from build123d import *
from build123d import SkipClean  # not in build123d's __all__

# Parameters (mm, degrees)
F1_DEPTH = 51
F2_DEPTH = 90


with BuildPart() as f1:
    # F0 (on Front) → F1 (new body)
    with BuildSketch(Plane.XZ):
        with BuildLine():
            Line((1.45, 0.9), (2.0621590627, 0.9))
            ThreePointArc((2.0621590627, 0.9), (1.5909902577, 1.5909902577), (0.9, 2.0621590627))
            Line((0.9, 2.0621590627), (0.9, 1.45))
            Line((0.9, 1.45), (0, 1.45))
            Line((0, 1.45), (-0.9, 1.45))
            Line((-0.9, 1.45), (-0.9, 2.0621590627))
            ThreePointArc((-0.9, 2.0621590627), (-1.5909902577, 1.5909902577), (-2.0621590627, 0.9))
            Line((-2.0621590627, 0.9), (-1.45, 0.9))
            Line((-1.45, 0.9), (-1.45, 0))
            Line((-1.45, 0), (-1.45, -0.9))
            Line((-1.45, -0.9), (-2.0621590627, -0.9))
            ThreePointArc((-2.0621590627, -0.9), (-1.5909902577, -1.5909902577), (-0.9, -2.0621590627))
            Line((-0.9, -2.0621590627), (-0.9, -1.45))
            Line((-0.9, -1.45), (0, -1.45))
            Line((0, -1.45), (0.9, -1.45))
            Line((0.9, -1.45), (0.9, -2.0621590627))
            ThreePointArc((0.9, -2.0621590627), (1.5909902577, -1.5909902577), (2.0621590627, -0.9))
            Line((2.0621590627, -0.9), (1.45, -0.9))
            Line((1.45, -0.9), (1.45, 0))
            Line((1.45, 0), (1.45, 0.9))
        make_face()
    extrude(amount=F1_DEPTH)

    # F0 (on Front) → F2 (join)
    with BuildSketch(Plane.XZ):
        with BuildLine():
            Line((1.45, 0.9), (2.0621590627, 0.9))
            ThreePointArc((2.0621590627, 0.9), (1.5909902577, 1.5909902577), (0.9, 2.0621590627))
            Line((0.9, 2.0621590627), (0.9, 1.45))
            Line((0.9, 1.45), (0, 1.45))
            Line((0, 1.45), (-0.9, 1.45))
            Line((-0.9, 1.45), (-0.9, 2.0621590627))
            ThreePointArc((-0.9, 2.0621590627), (-1.5909902577, 1.5909902577), (-2.0621590627, 0.9))
            Line((-2.0621590627, 0.9), (-1.45, 0.9))
            Line((-1.45, 0.9), (-1.45, 0))
            Line((-1.45, 0), (-1.45, -0.9))
            Line((-1.45, -0.9), (-2.0621590627, -0.9))
            ThreePointArc((-2.0621590627, -0.9), (-1.5909902577, -1.5909902577), (-0.9, -2.0621590627))
            Line((-0.9, -2.0621590627), (-0.9, -1.45))
            Line((-0.9, -1.45), (0, -1.45))
            Line((0, -1.45), (0.9, -1.45))
            Line((0.9, -1.45), (0.9, -2.0621590627))
            ThreePointArc((0.9, -2.0621590627), (1.5909902577, -1.5909902577), (2.0621590627, -0.9))
            Line((2.0621590627, -0.9), (1.45, -0.9))
            Line((1.45, -0.9), (1.45, 0))
            Line((1.45, 0), (1.45, 0.9))
        make_face()
        with BuildLine():
            Line((0.9, 1.45), (0.9, 2.0621590627))
            ThreePointArc((0.9, 2.0621590627), (0.4596966983, 2.2025392041), (0, 2.25))
            ThreePointArc((0, 2.25), (-0.4596966983, 2.2025392041), (-0.9, 2.0621590627))
            Line((-0.9, 2.0621590627), (-0.9, 1.45))
            Line((-0.9, 1.45), (0, 1.45))
            Line((0, 1.45), (0.9, 1.45))
        make_face()
        with BuildLine():
            Line((-1.45, 0.9), (-2.0621590627, 0.9))
            ThreePointArc((-2.0621590627, 0.9), (-2.2025392041, 0.4596966983), (-2.25, 0))
            ThreePointArc((-2.25, 0), (-2.2025392041, -0.4596966983), (-2.0621590627, -0.9))
            Line((-2.0621590627, -0.9), (-1.45, -0.9))
            Line((-1.45, -0.9), (-1.45, 0))
            Line((-1.45, 0), (-1.45, 0.9))
        make_face()
        with BuildLine():
            ThreePointArc((0, -2.25), (0.4596966983, -2.2025392041), (0.9, -2.0621590627))
            Line((0.9, -2.0621590627), (0.9, -1.45))
            Line((0.9, -1.45), (0, -1.45))
            Line((0, -1.45), (-0.9, -1.45))
            Line((-0.9, -1.45), (-0.9, -2.0621590627))
            ThreePointArc((-0.9, -2.0621590627), (-0.4596966983, -2.2025392041), (0, -2.25))
        make_face()
        with BuildLine():
            ThreePointArc((2.0621590627, -0.9), (2.2025392041, -0.4596966983), (2.25, 0))
            ThreePointArc((2.25, 0), (2.2025392041, 0.4596966983), (2.0621590627, 0.9))
            Line((2.0621590627, 0.9), (1.45, 0.9))
            Line((1.45, 0.9), (1.45, 0))
            Line((1.45, 0), (1.45, -0.9))
            Line((1.45, -0.9), (2.0621590627, -0.9))
        make_face()
    with SkipClean():  # cleaning this boolean's faces spoils the solid; the shape is the same uncleaned
        extrude(amount=-F2_DEPTH)


solid = f1.part
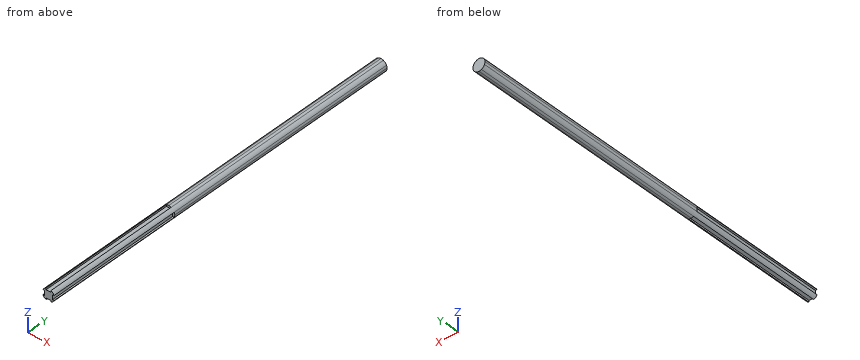
Read the model definition and answer for the solid it produces. Units are mm, in the model's axes. Coordinates: 2 decimals unless noted, no trailing zeros. Order: outer loops, then holes, each group sorted by start corner. A loop starts at its lowest first (then second) coordinate and runs counter-clockwise, first axis right, second up. Notation, with made-up numbers: (44.25, -15.5) -> (69.25, -15.5) arc R32 cw to (69.25, 17.5) -> close; hole circle Ø6 at (43, -18). An arc over 180 degrees is marked (long way). Answer as a JSON object with one key per item and string values.
1) A cutting plane is placed at A-A, the plane y = -13. Determine the outline of the cut face in (x, z), plus the area to 3 significant figures.
Model answer:
{"outline": "(-2.06, -0.9) arc R2.25 ccw to (-0.9, -2.06) -> (-0.9, -1.45) -> (0.9, -1.45) -> (0.9, -2.06) arc R2.25 ccw to (2.06, -0.9) -> (1.45, -0.9) -> (1.45, 0.9) -> (2.06, 0.9) arc R2.25 ccw to (0.9, 2.06) -> (0.9, 1.45) -> (-0.9, 1.45) -> (-0.9, 2.06) arc R2.25 ccw to (-2.06, 0.9) -> (-1.45, 0.9) -> (-1.45, -0.9) -> close", "area": "10.6 mm²"}
2) A cutting plane is placed at B-B, the plane y = 16. Determine the outline of the cut face in (x, z).
Model answer:
{"outline": "circle Ø4.5 at (0, 0)"}
3) Each of these flat-tipped pins is pushed along its axis until it touches: pin 1 (1.5 mm diameter, centred on y = -4.5, z = 1.5, fed in from -X); pin 2 (0.9 mm diameter, centred on y = -15.5, z = 0, fed in from -X); pin 3 (0.9 mm diameter, centred on y = -33, z = -0.5, fed in from +X). Where does it stop, or does it pass through?
Model answer:
{"pin 1": "stops at x = -2.06", "pin 2": "stops at x = -1.45", "pin 3": "stops at x = 2.06"}
4) Consider line 1 along Y through (x, z) = (0.8, 1.65); line 2 along X through (y, z) = (-21.5, -0.7); line 3 along Z through (x, y) = (-0.2, 63.5). Determine where each line is inside the solid, lowest interval first. Write a range as from..to.
Model answer:
{"line 1": "y = 0..90", "line 2": "x = -1.45..1.45", "line 3": "z = -2.24..2.24"}
